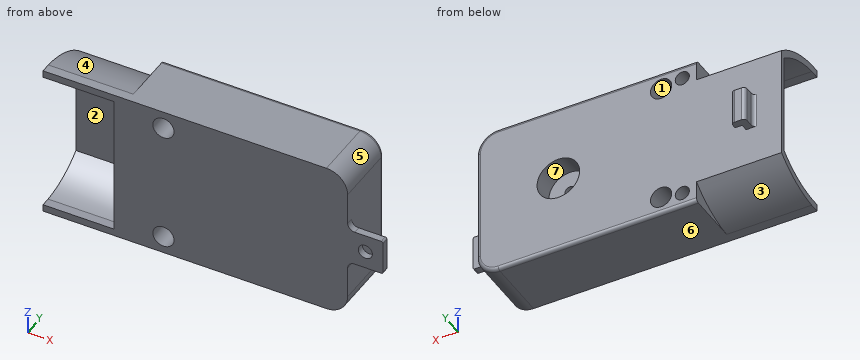
```python
from build123d import *

# Parameters (mm, degrees)
BOSS_EXTRUDE2_DEPTH = 9
SKETCH4_W           = 5
SKETCH4_H           = 1
BOSS_EXTRUDE3_DEPTH = 5
SKETCH5_R           = 1
CUT_EXTRUDE1_DEPTH  = 5
FILLET1_R           = 1
FILLET2_R           = 1
FILLET3_R           = 3
FILLET4_R           = 3
BOSS_EXTRUDE4_DEPTH = 12
FILLET5_R           = 0.5
FILLET6_R           = 0.25
SKETCH8_R           = 3
CUT_EXTRUDE3_DEPTH  = 3
SKETCH9_R           = 0.75
CUT_EXTRUDE4_DEPTH  = 3
SKETCH10_R          = 1.5
CUT_EXTRUDE7_DEPTH  = 44.13930922
SKETCH12_R          = 1
CUT_EXTRUDE8_DEPTH  = 5
SKETCH13_W          = 1
SKETCH13_H          = 5
BOSS_EXTRUDE5_DEPTH = 2
SKETCH14_W          = 5
SKETCH14_H          = 1
BOSS_EXTRUDE6_DEPTH = 1
FILLET7_R           = 0.5
FILLET8_R           = 0.5
FILLET9_R           = 0.5
CUT_EXTRUDE9_DEPTH  = 10


with BuildPart() as part:
    # Sketch2 → Boss-Extrude2 (new body)
    with BuildSketch(Plane(origin=(0, 0, 0), x_dir=(1, 0, 0), z_dir=(0, 1, 0))):
        Polygon((0, 11), (31, 11), (31, 13.5), (31, 22), (0, 22), align=None)
        Polygon((31, 8.5), (31, 11), (0, 11), (0, 0), (31, 0), align=None)
    extrude(amount=BOSS_EXTRUDE2_DEPTH)

    # Sketch4 → Boss-Extrude3 (add)
    with BuildSketch(Plane(origin=(31, 0, 0), x_dir=(0, 0, -1), z_dir=(1, 0, 0))):
        with Locations((11, 0.5)):
            Rectangle(SKETCH4_W, SKETCH4_H)
    extrude(amount=BOSS_EXTRUDE3_DEPTH)

    # Sketch5 → Cut-Extrude1 (cut)
    with BuildSketch(Plane(origin=(0, 1, 0), x_dir=(1, 0, 0), z_dir=(0, 1, 0))):
        with Locations(Location((33.5, 11, 0), (0, 0, 270))):
            Circle(SKETCH5_R)
    extrude(amount=-CUT_EXTRUDE1_DEPTH, mode=Mode.SUBTRACT)

    # Fillet1
    fillet1_edges = [part.edges().sort_by_distance(p)[0] for p in [
        (31, 0.5, -8.5),
    ]]
    fillet(fillet1_edges, radius=FILLET1_R)

    # Fillet2
    fillet2_edges = [part.edges().sort_by_distance(p)[0] for p in [
        (31, 0.5, -13.5),
    ]]
    fillet(fillet2_edges, radius=FILLET2_R)

    # Fillet3
    fillet3_edges = [part.edges().sort_by_distance(p)[0] for p in [
        (31, 4.5, 0),
    ]]
    fillet(fillet3_edges, radius=FILLET3_R)

    # Fillet4
    fillet4_edges = [part.edges().sort_by_distance(p)[0] for p in [
        (31, 4.5, -22),
    ]]
    fillet(fillet4_edges, radius=FILLET4_R)

    # Sketch6 → Boss-Extrude4 (add)
    with BuildSketch(Plane.ZY):
        with BuildLine():
            Line((-22, 0), (-11, 0))
            Line((-11, 0), (-11, 9))
            Line((-11, 9), (-19, 9))
            ThreePointArc((-19, 9), (-21.121122912, 5.415884648), (-22, 1.344936316))
            Line((-22, 1.344936316), (-22, 0))
        make_face()
        with BuildLine():
            Line((-11, 9), (-11, 0))
            Line((-11, 0), (0, 0))
            Line((0, 0), (0, 1.344936316))
            ThreePointArc((0, 1.344936316), (-0.878877088, 5.415884648), (-3, 9))
            Line((-3, 9), (-11, 9))
        make_face()
    extrude(amount=BOSS_EXTRUDE4_DEPTH)

    # Fillet5
    fillet5_edges = [part.edges().sort_by_distance(p)[0] for p in [
        (14, 9, -22),
        (30.121320344, 9, -21.121320344),
        (31, 9, -11),
        (30.121320344, 9, -0.878679656),
        (14, 9, 0),
    ]]
    fillet(fillet5_edges, radius=FILLET5_R)

    # Fillet6
    fillet6_edges = [part.edges().sort_by_distance(p)[0] for p in [
        (36, 0.5, -13.5),
        (36, 0.5, -8.5),
    ]]
    fillet(fillet6_edges, radius=FILLET6_R)

    # Sketch8 → Cut-Extrude3 (cut)
    with BuildSketch(Plane(origin=(0, 9, 0), x_dir=(1, 0, 0), z_dir=(0, 1, 0))):
        with Locations(Location((19.5, 11, 0), (0, 0, 270))):
            Circle(SKETCH8_R)
    extrude(amount=-CUT_EXTRUDE3_DEPTH, mode=Mode.SUBTRACT)

    # Sketch9 → Cut-Extrude4 (cut)
    with BuildSketch(Plane(origin=(0, 6, 0), x_dir=(1, 0, 0), z_dir=(0, 1, 0))):
        with Locations(Location((19.5, 11, 0), (0, 0, 270))):
            Circle(SKETCH9_R)
    extrude(amount=-CUT_EXTRUDE4_DEPTH, mode=Mode.SUBTRACT)

    # Sketch10 → Cut-Extrude7 (cut, through all)
    with BuildSketch(Plane(origin=(0, 9, 0), x_dir=(1, 0, 0), z_dir=(0, 1, 0))):
        with Locations(Location((5, 19.5, 0), (0, 0, 90))):
            Circle(SKETCH10_R)
        with Locations(Location((5, 2.5, 0), (0, 0, 270))):
            Circle(SKETCH10_R)
    extrude(amount=-CUT_EXTRUDE7_DEPTH, mode=Mode.SUBTRACT)

    # Sketch12 → Cut-Extrude8 (cut)
    with BuildSketch(Plane(origin=(0, 9, 0), x_dir=(1, 0, 0), z_dir=(0, 1, 0))):
        with Locations(Location((2, 2, 0), (0, 0, 270))):
            Circle(SKETCH12_R)
        with Locations(Location((2, 20, 0), (0, 0, 270))):
            Circle(SKETCH12_R)
    extrude(amount=-CUT_EXTRUDE8_DEPTH, mode=Mode.SUBTRACT)

    # Sketch13 → Boss-Extrude5 (add)
    with BuildSketch(Plane(origin=(0, 9, 0), x_dir=(1, 0, 0), z_dir=(0, 1, 0))):
        with Locations((-7.5, 11)):
            Rectangle(SKETCH13_W, SKETCH13_H)
    extrude(amount=BOSS_EXTRUDE5_DEPTH)

    # Sketch14 → Boss-Extrude6 (add)
    with BuildSketch(Plane(origin=(-7, 0, 0), x_dir=(0, 0, -1), z_dir=(1, 0, 0))):
        with Locations((11, 10.5)):
            Rectangle(SKETCH14_W, SKETCH14_H)
    extrude(amount=BOSS_EXTRUDE6_DEPTH)

    # Fillet7
    fillet7_edges = [part.edges().sort_by_distance(p)[0] for p in [
        (-8, 11, -11),
    ]]
    fillet(fillet7_edges, radius=FILLET7_R)

    # Fillet8
    fillet8_edges = [part.edges().sort_by_distance(p)[0] for p in [
        (-8, 9, -11),
    ]]
    fillet(fillet8_edges, radius=FILLET8_R)

    # Fillet9
    fillet9_edges = [part.edges().sort_by_distance(p)[0] for p in [
        (-6, 11, -11),
    ]]
    fillet(fillet9_edges, radius=FILLET9_R)

    # Sketch16 → Cut-Extrude9 (cut)
    with BuildSketch(Plane.ZY.offset(12)):
        with BuildLine():
            Line((-18.232108037, 8.359420628), (-3.767891963, 8.359420628))
            ThreePointArc((-3.767891963, 8.359420628), (-1.809932353, 5.051006457), (-0.998661194, 1.293207997))
            Line((-0.998661194, 1.293207997), (-0.998661194, 0))
            Line((-0.998661194, 0), (-21, 0))
            Line((-21, 0), (-21.001338806, 1.293207997))
            ThreePointArc((-21.001338806, 1.293207997), (-20.190067647, 5.051006457), (-18.232108037, 8.359420628))
        make_face()
    extrude(amount=-CUT_EXTRUDE9_DEPTH, mode=Mode.SUBTRACT)


solid = part.part
```
The model under review builds one solid part; all positions refer to its coordinate system, in mm. Face numbers are marked on the shaded views. A direction names the side the tool comes from. Round coordinates to 2 decimals unless told otherwise and drop trailing zeros. Loops run counter-clockwise (first coordinate to the right, second up) from the corner with the lowest first, then second, coordinate; pieces in that order, holes last. Notation, with made-up numbers: (0, 41.5) - (51, 41.5) arc R21 ccw to (51, 73.5) - close; hole circle Ø10 at (30.5, 45.25). An arc over 180 degrees is marked (long way). Write each question's results on one line, items separated by ' | '. Start each with the question number.
Q1. Take a section at B-B on y = 7.5. Give the boundary of the cut face in (x, z).
Q2. Tool access review of the marked faces 1, 2, 3 and 4: name each direction out of +Z, -Z, +X, -X, +Y, -Y from which nothing blocks a thin tool from reaching the whole face with its end or side.
Q3. Wall thickness on line 1 along X through (y, z) = (0.5, -11); line 2 along Z through (x, y) = (-4.5, 1); line 3 along X through (y, z) = (7.15, -11): over which ranges is each line inside the solid? List them lowest first. Write a range as [from, to].
Q4. Take a section at C-C on x = 14. Give the boundary of the cut face in (y, z), plus the area to 3 significant figures.
Q5. Insertion check: P1, Ø1.5, axis at y = 5.5, z = -5.5, coming from the -X side; P2, Ø5, axis at x = 5, z = -2.5, coming from the +Y side; P3, Ø0.8, axis at x = -6.5, z = -11.5, coming from the -Y side. Each pin has a flat end and moves straight along its axis. Give the tip position at first contact, or say it passes through.
Q6. Draft analysis for pull direction X (two halves, no side actions). For the marked faces 5, 6 and 7, state which applies: pulls with the +X half, pulls with the -X half, needs draft (parallel to the pull), parting line crosses it, or undercut.
Q7. Take a section at D-D on z = -15.5. Give the boundary of the cut face in (x, y), plus the area to 3 significant figures.
Q8. Take a section at A-A on x = 5. Give the boundary of the cut face in (y, z), plus the area to 3 significant figures.
Data:
1) outline: (-12, -20.08) - (0, -20.08) - (0, -22) - (28, -22) arc R3 ccw to (31, -19) - (31, -3) arc R3 ccw to (28, 0) - (0, 0) - (0, -1.92) - (-12, -1.92) - (-12, -3.11) - (-2, -3.11) - (-2, -18.89) - (-12, -18.89) - close; hole circle Ø2 at (2, -20); hole circle Ø2 at (2, -2); hole circle Ø3 at (5, -19.5); hole circle Ø3 at (5, -2.5); hole circle Ø6 at (19.5, -11)
2) face 1: +Y, -Y | face 2: -X, -Y | face 3: -Z, -X, +Y | face 4: +Z, -X, +Y
3) line 1: x = [-2, 32.5], [34.5, 36] | line 2: z = [-22, -21], [-1, 0] | line 3: x = [-2, 16.5], [22.5, 31]
4) outline: (0, -22) - (8.5, -22) arc R0.5 ccw to (9, -21.5) - (9, -0.5) arc R0.5 ccw to (8.5, 0) - (0, 0) - close | area: 198 mm²
5) P1: stops at x = -2 | P2: stops at y = 9 | P3: stops at y = 8.36
6) face 5: pulls with the +X half | face 6: needs draft | face 7: undercut
7) outline: (-12, 8.36) - (-2, 8.36) - (-2, 0) - (31, 0) - (31, 8.5) arc R0.5 ccw to (30.5, 9) - (-12, 9) - close | area: 303 mm²
8) outline: (0, -22) - (8.5, -22) arc R0.5 ccw to (9, -21.5) - (9, -21) - (0, -21) - close; (0, -18) - (9, -18) - (9, -4) - (0, -4) - close; (0, -1) - (9, -1) - (9, -0.5) arc R0.5 ccw to (8.5, 0) - (0, 0) - close | area: 144 mm²
